Work out the finished part from the listing and answer in its coordinate system (mm). A direction names the side the tool comes from. Coordinates: 2 decimals unless noted, no trailing zeros. Loops run counter-clockwise (first coordinate to the right, second up) from the corner with the lowest first, then second, coordinate; pieces in that order, holes last. Notation, with made-up numbers: (-19, 64.5) - (21, 64.5) arc R17 cw to (21, 89.5) - close; hole circle Ø9 at (79.5, 67.5). An arc over 180 degrees is marked (long way). Write each question's results on one line, items separated by ' | '. Start each with the question number.
1. A cutting plane is placed at A-A on y = 599.5. Determine the outline of the cut face in (x, z), then the cut area to 3 significant figures.
2. Which of the six approach directions +Z, -Z, +X, -X, +Y, -Y give full straight-line access (tool end or side, diameter ignored) to faces 4 (the flat face through (451, 889, 875)), 5 (the flat face through (25.4, 438, 376)), 6 (the flat face through (464, 914.4, 476))?
3. Find the intervals of material crossed by line 1 along X through (y, z) = (787.5, 180.5); line 2 along Z through (x, y) = (263, 51); line 3 along Y through (x, z) = (368, 921.5), in increasing order. Write a range as [from, to].
4. Each of these flat-tipped pins is pushed along its axis until it touches: P1, Ø10, axis at x = 249.5, y = 171, coming from the -Z side; P2, Ø4, axis at x = 652.5, y = 127.5, coming from the +Z side. Where does it stop, or does it pass through?
5. A cutting plane is placed at B-B on z = 872. Determine the outline of the cut face in (x, y).
6. Determine the mould class of faces 1 (the flat face through (0, 464, 476)), 2 (the flat face through (463, 451, 787.4)), 3 (the flat face through (455, 0, 766)) for opening direction X: released by +X, released by -X, zero draft, split by the parting line, or undercut.
7. A cutting plane is placed at C-C on x = 82. Determine the outline of the cut face in (y, z), then the cut area to 3 significant figures.
from build123d import *

# Parameters (mm, degrees)
F1_DEPTH = 914.4
F2_W     = 889
F2_H     = 25.4
F3_DEPTH = 889
F4_DEPTH = 50.8


with BuildPart() as f1:
    # F0 (on Top) → F1 (new body)
    with BuildSketch(Plane.XY):
        Polygon((889, 914.4), (0, 914.4), (0, 25.4), (0, 0), (25.4, 0), (25.4, 25.4), (25.4, 889), (889, 889), (889, 25.4), (889, 0), (914.4, 0), (914.4, 889), (914.4, 914.4), align=None)
    extrude(amount=F1_DEPTH)

    # F2 (on face) → F3 (join)
    with BuildSketch(Plane(origin=(889, 0, 0), x_dir=(0, -1, 0), z_dir=(-1, 0, 0))):
        with Locations((-444.5, 774.7)):
            Rectangle(F2_W, F2_H)
    extrude(amount=F3_DEPTH)

    # F4 (add): a face of the model
    f4_faces = [f1.faces().sort_by_distance(p)[0] for p in [
        (457.2, 901.4684311857, 914.4),
    ]]
    extrude(f4_faces, amount=F4_DEPTH)


solid = f1.part
Values:
1) outline: (0, 0) - (25.4, 0) - (25.4, 762) - (889, 762) - (889, 0) - (914.4, 0) - (914.4, 965.2) - (889, 965.2) - (889, 787.4) - (25.4, 787.4) - (25.4, 965.2) - (0, 965.2) - close | area: 71,000 mm^2
2) face 4: +Z, -Y | face 5: -Z, -Y | face 6: +Z, -Z, +X, -X, +Y
3) line 1: [0, 25.4], [889, 914.4] | line 2: [762, 787.4] | line 3: [889, 914.4]
4) P1: z = 762 | P2: z = 787.4
5) outline: (0, 0) - (25.4, 0) - (25.4, 889) - (889, 889) - (889, 0) - (914.4, 0) - (914.4, 914.4) - (0, 914.4) - close
6) face 1: released by -X | face 2: undercut | face 3: zero draft
7) outline: (0, 762) - (889, 762) - (889, 0) - (914.4, 0) - (914.4, 965.2) - (889, 965.2) - (889, 787.4) - (0, 787.4) - close | area: 47,100 mm^2
